from build123d import *

# Parameters (mm, degrees)
F0_W      = 50.8
F0_H      = 50.8
F1_DEPTH  = 38.1
F2_T      = -3.81
F10_W     = 12.7
F10_H     = 12.7
F11_DEPTH = 25.4
F12_W     = 12.7
F12_H     = 12.7
F13_DEPTH = 25.4
F14_W     = 8.89
F14_H     = 8.89
F15_DEPTH = 25.4


# Not quite as in the source:
# - the program builds the solid bodies; features that only make, move or delete a surface that nothing else refers to are left out


with BuildPart() as f1:
    # F0 (on Top) → F1 (new body)
    with BuildSketch(Plane.XY):
        with Locations((0.1272018999, -1.6994403997)):
            Rectangle(F0_W, F0_H)
    extrude(amount=F1_DEPTH)

    # F2
    f2_openings = [f1.faces().sort_by_distance(p)[0] for p in [
        (0.127202, -1.69944, 38.1),
        (0.127202, -1.69944, 0),
    ]]
    offset(amount=F2_T, openings=f2_openings)

    # F10 (on face) → F11 (cut)
    with BuildSketch(Plane.YZ.offset(25.5272018999)):
        with Locations((-1.6994403997, 19.05)):
            Rectangle(F10_W, F10_H)
    extrude(amount=-F11_DEPTH, mode=Mode.SUBTRACT)

    # F12 (on face) → F13 (cut)
    with BuildSketch(Plane(origin=(-25.2727981001, 0, 0), x_dir=(0, -1, 0), z_dir=(-1, 0, 0))):
        with Locations((1.6994403997, 19.05)):
            Rectangle(F12_W, F12_H)
    extrude(amount=-F13_DEPTH, mode=Mode.SUBTRACT)

    # F14 (on face) → F15 (cut)
    with BuildSketch(Plane.XZ.offset(27.0994403997)):
        with Locations((16.0022018999, 23.495)):
            Rectangle(F14_W, F14_H)
        with Locations((-15.7477981001, 23.495)):
            Rectangle(F14_W, F14_H)
    extrude(amount=-F15_DEPTH, mode=Mode.SUBTRACT)


solid = f1.part
CAD build for the part. Positions are in the model's coordinates, mm. A direction names the side the tool comes from. Round coordinates to 2 decimals unless told otherwise and drop trailing zeros. Write each loop counter-clockwise with the first axis right and the second up, starting at its lowest first coordinate (ties: lowest second). Pieces come first, ordered by that corner, then holes. Notation, with made-up numbers: M 31,31 L 64,31 A18 cw 64,49 Z; hole C 68.25,-37 d11. An arc over 180 degrees is marked long. Use a Markdown table: item, result. Add a question column.
1. Pull direction Y, two halves, no side cores. Call faces 6 (the face through (0, 19.891, 19)), 7 (the face through (22, -1, 38.1)), 8 (the face through (0, -27.099, 19)): released by +Y, released by -Y, zero draft, split by the parting line, or undercut.
2. Slice it at A-A on x = -14.5. Give the cut face in (y, z).
3. Slice it at D-D on x = 10.5. Give the cut face in (y, z), then the cut area to 3 significant figures.
4. Drill centre lines: probe 1 along Y at (x, z) = (16, 15); probe 2 along X at (y, z) = (-22, 25); probe 3 along Y at (x, z) = (-19, 25). Where is each one in solid material? Low to high.
5. 3-axis set-ups, long thin cutter, end or side, ignore diameter. For faces 1 (the face through (-25.273, -2, 27)), 2 (the face through (0, 23.701, 19)), 3 (the face through (-23, -2, 25.4)), 4 (the face through (-16, -25, 19.05)), 5 (the face through (21.717, -2, 27)): which of +Z, -Z, +X, -X, +Y, -Y reach the whole face in a straight line?
6. Slice it at B-B on y = -12.5. Give the cut face in (x, z).
7. Slice it at C-C on z = 10.5. Give the cut face in (x, y), then the cut area to 3 significant figures.
8. Flat gauge pins, fed straight in: P1, Ø12, axis at x = -14.5, y = 1, coming from the +Z side; P2, Ø1.1, axis at x = 24, y = -1, coming from the -Z side. Where does each tip first touch, or does it go through?
Reply:
| question | item | result |
|---|---|---|
| 1 | face 6 | undercut |
| 1 | face 7 | zero draft |
| 1 | face 8 | released by -Y |
| 2 | outline | M -27.1,0 L -23.29,0 L -23.29,19.05 L -27.1,19.05 Z; M -27.1,27.94 L -23.29,27.94 L -23.29,38.1 L -27.1,38.1 Z; M 19.89,0 L 23.7,0 L 23.7,38.1 L 19.89,38.1 Z |
| 3 | outline | M -27.1,0 L -23.29,0 L -23.29,38.1 L -27.1,38.1 Z; M 19.89,0 L 23.7,0 L 23.7,38.1 L 19.89,38.1 Z |
| 3 | area | 290 mm^2 |
| 4 | probe 1 | y = -27.1 to -23.29, 19.89 to 23.7 |
| 4 | probe 2 | x = -25.27 to -21.46, 21.72 to 25.53 |
| 4 | probe 3 | y = 19.89 to 23.7 |
| 5 | face 1 | +Z, -Z, -X, +Y, -Y |
| 5 | face 2 | +Z, -Z, +X, -X, +Y |
| 5 | face 3 | +X, -X |
| 5 | face 4 | -Y |
| 5 | face 5 | +Z, -Z |
| 6 | outline | M -25.27,0 L -21.46,0 L -21.46,38.1 L -25.27,38.1 Z; M 21.72,0 L 25.53,0 L 25.53,38.1 L 21.72,38.1 Z |
| 7 | outline | M -25.27,-27.1 L 25.53,-27.1 L 25.53,23.7 L -25.27,23.7 Z; hole M -21.46,-23.29 L 21.72,-23.29 L 21.72,19.89 L -21.46,19.89 Z |
| 7 | area | 716 mm^2 |
| 8 | P1 | passes through |
| 8 | P2 | stops at z = 0 |
